Geometry: final body of the model. Coordinates: model frame, mm. Face numbers are marked on the shaded views. A direction names the side the tool comes from. Give positions to 0.01 mm unless a question says otherwise; leave off trailing zeros. Loops run counter-clockwise (first coordinate to the right, second up) from the corner with the lowest first, then second, coordinate; pieces in that order, holes last. Notation, with made-up numbers: (74.5, 74) - (88.5, 74) arc R16 cw to (88.5, 96) - close; hole circle Ø7 at (32.25, 32.25). An arc over 180 degrees is marked (long way). Use one line per item in the form item = value.
```python
from build123d import *

# Parameters (mm, degrees)
F0_W      = 50
F0_H      = 30
F1_DEPTH  = 8
F2_R      = 2.85
F3_DEPTH  = 8
F4_R      = 1.5
F5_DEPTH  = 3
F6_DEPTH  = 4
F7_DEPTH  = 1
F8_R      = 6.75
F9_DEPTH  = 2
F11_DEPTH = 6


with BuildPart() as f1:
    # F0 (on Top) → F1 (new body)
    with BuildSketch(Plane.XY):
        with Locations((25, 15)):
            Rectangle(F0_W, F0_H)
    extrude(amount=F1_DEPTH)

    # F2 (on face) → F3 (cut)
    with BuildSketch(Plane.XY.offset(8)):
        with Locations((41, 19)):
            Circle(F2_R)
        with Locations((9, 19)):
            Circle(F2_R)
    extrude(amount=-F3_DEPTH, mode=Mode.SUBTRACT)

    # F4 (on face) → F5 (cut)
    with BuildSketch(Plane.XZ):
        with Locations((5, 4)):
            Circle(F4_R)
        with Locations((45, 4)):
            Circle(F4_R)
    extrude(amount=-F5_DEPTH, mode=Mode.SUBTRACT)

    # F4 (on face) → F6 (cut)
    with BuildSketch(Plane.XZ):
        Polygon((22.15, 0.75), (22.15, 0), (27.85, 0), (27.85, 0.75), (25.85, 0.75), (25.85, 2.75), (27.85, 2.75), (27.85, 6.25), (25.85, 6.25), (25.85, 7.25), (27.85, 7.25), (27.85, 8), (22.15, 8), (22.15, 7.25), (24.15, 7.25), (24.15, 6.25), (22.15, 6.25), (22.15, 2.75), (24.15, 2.75), (24.15, 0.75), align=None)
    extrude(amount=-F6_DEPTH, mode=Mode.SUBTRACT)

    # F4 (on face) → F7 (cut)
    with BuildSketch(Plane.XZ):
        Polygon((19.15, 8), (19.15, 0), (22.15, 0), (22.15, 0.75), (24.15, 0.75), (24.15, 2.75), (22.15, 2.75), (22.15, 6.25), (24.15, 6.25), (24.15, 7.25), (22.15, 7.25), (22.15, 8), align=None)
        Polygon((27.85, 0.75), (27.85, 0), (30.85, 0), (30.85, 8), (27.85, 8), (27.85, 7.25), (25.85, 7.25), (25.85, 6.25), (27.85, 6.25), (27.85, 2.75), (25.85, 2.75), (25.85, 0.75), align=None)
    extrude(amount=-F7_DEPTH, mode=Mode.SUBTRACT)

    # F8 (on face) → F9 (cut)
    with BuildSketch(Plane(origin=(0, 0, 0), x_dir=(1, 0, 0), z_dir=(0, 0, -1))):
        with Locations((25, -19)):
            Circle(F8_R)
    extrude(amount=-F9_DEPTH, mode=Mode.SUBTRACT)

    # F10 (on face) → F11 (cut)
    with BuildSketch(Plane(origin=(0, 0, 2), x_dir=(1, 0, 0), z_dir=(0, 0, -1))):
        Polygon((30.918031, -20.31412), (29.097077, -14.531895), (23.179046, -13.217775), (19.081969, -17.68588), (20.902923, -23.468105), (26.820954, -24.782225), align=None)
    extrude(amount=-F11_DEPTH, mode=Mode.SUBTRACT)


solid = f1.part
```
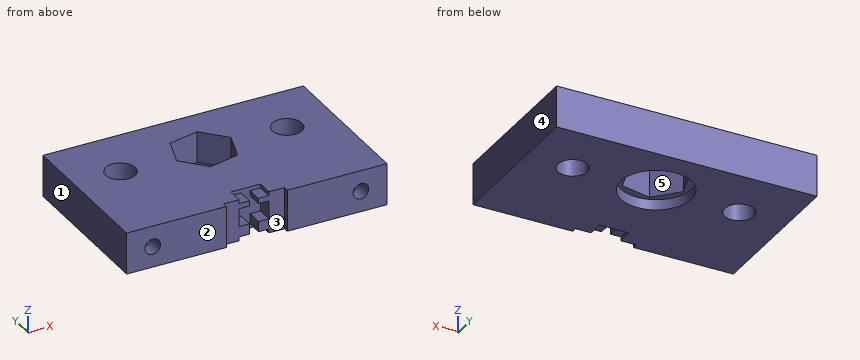
(1) Access query for the marked faces 4 and 5. Directions: +Z, -Z, +X, -X, +Y, -Y. A direction counts if a zero-diameter tool reaches every point of the face in a straight line with its end or side. Return the directions, or none.
Solution:
face_4 = +Z, -Z, +X, +Y, -Y
face_5 = +Z, -Z
(2) Material intervals for L1, parallel to Y at x = 41, z = 5.5; L2, parallel to X at y = 18.25, z = 5; L3, parallel to Y at x = 25, z = 1.45, sorted ascending. Write a range as from..to.
Solution:
L1 = 0..16.15, 21.85..30
L2 = 0..6.25, 11.75..19.26, 30.27..38.25, 43.75..50
L3 = 4..12.25, 25.75..30
(3) Cut plane B-B (y = 17). Return the cut outline in (x, z).
Solution:
outline = (0, 0) - (6.97, 0) - (6.97, 8) - (0, 8) - close; (11.03, 0) - (18.55, 0) - (18.55, 2) - (19.71, 2) - (19.71, 8) - (11.03, 8) - close; (29.87, 2) - (31.45, 2) - (31.45, 0) - (38.97, 0) - (38.97, 8) - (29.87, 8) - close; (43.03, 0) - (50, 0) - (50, 8) - (43.03, 8) - close
(4) Cut plane C-C (x = 25). Return the cut outline in (y, z), plus the area to 3 significant figures.
Solution:
outline = (4, 0) - (12.25, 0) - (12.25, 2) - (13.62, 2) - (13.62, 8) - (4, 8) - close; (24.38, 2) - (25.75, 2) - (25.75, 0) - (30, 0) - (30, 8) - (24.38, 8) - close
area = 116 mm2
(5) Pull-direction query (X, two-part tool) for the marked faces 1, 2 and 3; classes: released by +X, released by -X, zero draft, split by the parting line, or undercut.
Solution:
face_1 = released by -X
face_2 = zero draft
face_3 = undercut
(6) Cut plane D-D (x = 42.5). Return the cut outline in (y, z), plus the area to 3 significant figures.
Solution:
outline = (0, 0) - (16.58, 0) - (16.58, 8) - (0, 8) - close; (21.42, 0) - (30, 0) - (30, 8) - (21.42, 8) - close
area = 201 mm2
(7) Pin query (flat end, axial travel): P1, Ø4, axis at x = 28.5, z = 3.5, coming from the -Y side; P2, Ø1.6, axis at x = 23.5, y = 3, coming from the -Z side; P3, Ø0.6, axis at x = 27, y = 2.5, coming from the +Z side. Return the tip coordinate at first contact, or that it passes through.
Solution:
P1 = 1
P2 = 0.75
P3 = 7.25
(8) Cut plane A-A (z = 4). Return the cut outline in (x, y), plus the area to 3 significant figures.
Solution:
outline = (0, 0) - (3.5, 0) - (3.5, 3) - (6.5, 3) - (6.5, 0) - (19.15, 0) - (19.15, 1) - (22.15, 1) - (22.15, 4) - (27.85, 4) - (27.85, 1) - (30.85, 1) - (30.85, 0) - (43.5, 0) - (43.5, 3) - (46.5, 3) - (46.5, 0) - (50, 0) - (50, 30) - (0, 30) - close; hole circle Ø5.7 at (9, 19); hole (19.08, 17.69) - (23.18, 13.22) - (29.1, 14.53) - (30.92, 20.31) - (26.82, 24.78) - (20.9, 23.47) - close; hole circle Ø5.7 at (41, 19)
area = 1,310 mm2
